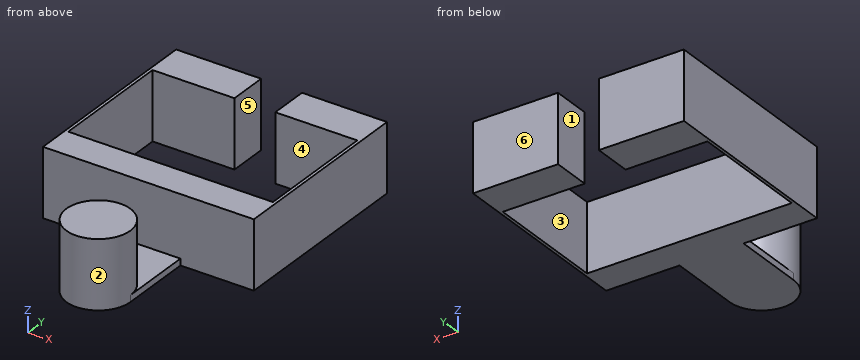
```python
from build123d import *

# Parameters (mm, degrees)
SKETCH1_R           = 9.913174659
BOSS_EXTRUDE1_DEPTH = 21.074744356
SKETCH2_W           = 19.826349318
SKETCH2_H           = 22.613174659
BOSS_EXTRUDE2_DEPTH = 2.024744356
SKETCH3_W           = 63.40856
SKETCH3_H           = 21.074744356
BOSS_EXTRUDE3_DEPTH = 10.014018179
SKETCH4_W           = 0.952402748
SKETCH4_H           = 21.074744356
BOSS_EXTRUDE4_DEPTH = 38.0746
SKETCH5_W           = 0.952402748
SKETCH5_H           = 21.074744356
BOSS_EXTRUDE5_DEPTH = 10.014018179
SKETCH6_W           = 21.074744356
SKETCH6_H           = 12.042842766
BOSS_EXTRUDE6_DEPTH = 25.37968
SKETCH6_3_W         = 21.074744356
SKETCH6_3_H         = 12.042842766
BOSS_EXTRUDE7_DEPTH = 0.952402748


with BuildPart() as part:
    # Sketch1 → Boss-Extrude1 (new body)
    with BuildSketch(Plane.XY):
        Circle(SKETCH1_R)
    extrude(amount=BOSS_EXTRUDE1_DEPTH)

    # Sketch2 → Boss-Extrude2 (add)
    with BuildSketch(Plane(origin=(0, 0, 0), x_dir=(-1, 0, 0), z_dir=(0, 0, -1))):
        with Locations((0, 11.30658733)):
            Rectangle(SKETCH2_W, SKETCH2_H)
    extrude(amount=-BOSS_EXTRUDE2_DEPTH)

    # Sketch3 → Boss-Extrude3 (add)
    with BuildSketch(Plane(origin=(0, 22.613174659, 0), x_dir=(1, 0, 0), z_dir=(0, 1, 0))):
        with Locations((0, -10.537372178)):
            Rectangle(SKETCH3_W, SKETCH3_H)
    extrude(amount=BOSS_EXTRUDE3_DEPTH)



with BuildPart() as body_2:
    # Sketch4 → Boss-Extrude4 (new body)
    with BuildSketch(Plane(origin=(0, 32.627192838, 0), x_dir=(1, 0, 0), z_dir=(0, 1, 0))):
        with Locations((32.180481374, -10.537372178)):
            Rectangle(SKETCH4_W, SKETCH4_H)
    boss_extrude4 = extrude(amount=BOSS_EXTRUDE4_DEPTH)


with BuildPart() as part_1:
    add(part.part)

    add(body_2.part)  # Boss-Extrude5 merges body 2
    # Sketch5 → Boss-Extrude5 (add)
    with BuildSketch(Plane.XZ.offset(-32.627192838)):
        with Locations((32.180481374, 10.537372178)):
            Rectangle(SKETCH5_W, SKETCH5_H)
    boss_extrude5 = extrude(amount=BOSS_EXTRUDE5_DEPTH)



with BuildPart() as body_2_2:
    # Sketch6 → Boss-Extrude6 (new body)
    with BuildSketch(Plane.ZY.offset(-31.70428)):
        with Locations((10.537372178, 76.723214221)):
            Rectangle(SKETCH6_W, SKETCH6_H)
    boss_extrude6 = extrude(amount=BOSS_EXTRUDE6_DEPTH)


with BuildPart() as part_2:
    add(part_1.part)

    add(body_2_2.part)  # Boss-Extrude7 merges body 2 2
    # Sketch6<3> → Boss-Extrude7 (add)
    with BuildSketch(Plane.ZY.offset(-31.70428)):
        with Locations((10.537372178, 76.723214221)):
            Rectangle(SKETCH6_3_W, SKETCH6_3_H)
    boss_extrude7 = extrude(amount=-BOSS_EXTRUDE7_DEPTH)

    # Mirror4: Boss-Extrude5 across plane
    add(boss_extrude5.mirror(Plane(origin=(0, 0, 0), x_dir=(0, 0, 1), z_dir=(1, 0, 0))))

    # Mirror5: Boss-Extrude4 across plane
    add(boss_extrude4.mirror(Plane(origin=(0, 0, 0), x_dir=(0, 0, 1), z_dir=(1, 0, 0))))

    # Mirror8: Boss-Extrude7 across plane
    add(boss_extrude7.mirror(Plane(origin=(0, 0, 0), x_dir=(0, 0, 1), z_dir=(1, 0, 0))))

    # Mirror9: Boss-Extrude6 across plane
    add(boss_extrude6.mirror(Plane(origin=(0, 0, 0), x_dir=(0, 0, 1), z_dir=(1, 0, 0))))


solid = part_2.part
```
The model under review builds one solid part; all positions refer to its coordinate system, in mm. Face numbers are marked on the shaded views. A direction names the side the tool comes from. Round coordinates to 2 decimals unless told otherwise and drop trailing zeros. Loops run counter-clockwise (first coordinate to the right, second up) from the corner with the lowest first, then second, coordinate; pieces in that order, holes last.
Item 1: Take a section at D-D (x = 0). Write out the cut boundary in (y, z).
Determined:
outline: (-9.91, 0) - (32.63, 0) - (32.63, 21.07) - (22.61, 21.07) - (22.61, 2.02) - (9.91, 2.02) - (9.91, 21.07) - (-9.91, 21.07) - close
Item 2: Take a section at A-A (y = 68.5). Write out the cut boundary in (x, z).
Determined:
outline: (-32.66, 0) - (-31.7, 0) - (-31.7, 21.07) - (-32.66, 21.07) - close; (31.7, 0) - (32.66, 0) - (32.66, 21.07) - (31.7, 21.07) - close
Item 3: For the marked faces 1, 2 and 3, list the 3-axis set-ups (+Z, -Z, +X, -X, +Y, -Y) from which the entire face can be reached by the end or side of a thin tool; tool diameter is ignored.
Determined:
face 1: +Z, -Z, +Y
face 2: +Z
face 3: +Z, -Z
Item 4: Take a section at C-C (x = 12). Write out the cut boundary in (y, z), then the cut area to 3 significant figures.
Determined:
outline: (22.61, 0) - (32.63, 0) - (32.63, 21.07) - (22.61, 21.07) - close; (70.7, 0) - (82.74, 0) - (82.74, 21.07) - (70.7, 21.07) - close
area: 465 mm2
Item 5: For line 1 (Y direction, x = -18, z = 2); line 2 (X direction, y = 49, z = 18); line 3 (Z direction, x = 8.5, y = 9), list the stretches that pass through material, from the lowest coordinate up.
Determined:
line 1: y = 22.61 to 32.63, 70.7 to 82.74
line 2: x = -32.66 to -31.7, 31.7 to 32.66
line 3: z = 0 to 2.02
Item 6: Take a section at B-B (z = 8). Write out the cut boundary in (x, y).
Determined:
outline: (-32.66, 22.61) - (32.66, 22.61) - (32.66, 82.74) - (6.32, 82.74) - (6.32, 70.7) - (31.7, 70.7) - (31.7, 32.63) - (-31.7, 32.63) - (-31.7, 70.7) - (-6.32, 70.7) - (-6.32, 82.74) - (-32.66, 82.74) - close; circle Ø19.83 at (0, 0)
Item 7: Mouldability with a two-part tool opening along Y and no side actions: class the marked faces 4, 5 and 6 as released by +Y, released by -Y, zero draft, split by the parting line, or undercut.
Determined:
face 4: undercut
face 5: zero draft
face 6: released by +Y
Item 8: Clearance check with flat-ended pins moving along their axes: pin 1 Ø10.5 at (x, z) = (25, 6.5) entering from -Y; pin 2 Ø1 at (y, z) = (22, 17) entering from +X; pin 3 Ø1.6 at (y, z) = (14.5, 0.5) entering from +X; pin 4 Ø0.6 at (y, z) = (7.5, 1.5) entering from -X. State where each tip first meets the part, or that it passes through.
Determined:
pin 1: stops at y = 22.61
pin 2: passes through
pin 3: stops at x = 9.91
pin 4: stops at x = -9.91
